For this review, take the finished solid that the model builds, in its own axes (mm). A direction names the side the tool comes from. Give positions to 0.01 mm unless a question says otherwise; leave off trailing zeros. Write each loop counter-clockwise with the first axis right and the second up, starting at its lowest first coordinate (ties: lowest second). Pieces come first, ordered by that corner, then holes. Notation, with made-up numbers: M 4,81 L 62,81 A17 cw 62,109 Z; hole C -38.5,-5.5 d8. An arc over 180 degrees is marked long. Answer as a JSON object with one key per item and string values. Group by question number.
```python
from build123d import *

# Parameters (mm, degrees)
SKETCH2_W                       = 25
SKETCH2_H                       = 130
SKETCH2_R                       = 5.1
SKETCH2_R_2                     = 7.5
BOSS_EXTRUDE1_DEPTH             = 6.35
TAP_DRILL_FOR_M3X0_5_TAP1_D     = 2.5
TAP_DRILL_FOR_M3X0_5_TAP1_DEPTH = 12.5
TAP_DRILL_FOR_M3X0_5_TAP1_TIP   = 0.751075774
BOSS_EXTRUDE2_DEPTH             = 6.35
F_1_4_CLEARANCE_HOLE1_D         = 6.7564
TAP_DRILL_FOR_M3X0_5_TAP2_D     = 2.5


with BuildPart() as part:
    # Sketch2 → Boss-Extrude1 (new body)
    with BuildSketch(Plane.XY):
        with Locations((0, 43.85)):
            Rectangle(SKETCH2_W, SKETCH2_H)
        Circle(SKETCH2_R, mode=Mode.SUBTRACT)
        with Locations((0, 25)):
            Circle(SKETCH2_R_2, mode=Mode.SUBTRACT)
        with Locations((0, 50)):
            Circle(SKETCH2_R_2, mode=Mode.SUBTRACT)
    extrude(amount=BOSS_EXTRUDE1_DEPTH)

    # Tap Drill for M3x0.5 Tap1
    with Locations(Plane.ZY.offset(12.5)):
        with Locations((3.175, 50), (3.175, 0), (3.175, 25)):
            Hole(TAP_DRILL_FOR_M3X0_5_TAP1_D / 2, depth=TAP_DRILL_FOR_M3X0_5_TAP1_DEPTH)
            with Locations((0, 0, -(TAP_DRILL_FOR_M3X0_5_TAP1_DEPTH + TAP_DRILL_FOR_M3X0_5_TAP1_TIP / 2))):  # 118° drill point
                Cone(0, TAP_DRILL_FOR_M3X0_5_TAP1_D / 2, TAP_DRILL_FOR_M3X0_5_TAP1_TIP, mode=Mode.SUBTRACT)

    # Sketch8 → Boss-Extrude2 (add)
    with BuildSketch(Plane(origin=(0, 0, 0), x_dir=(-1, 0, 0), z_dir=(0, 0, -1))):
        Polygon((12.5, 73.85), (22.5, 83.85), (22.5, 108.85), (12.5, 108.85), align=None)
    extrude(amount=-BOSS_EXTRUDE2_DEPTH)

    # 1/4 Clearance Hole1 (through all)
    with Locations(Plane.XY.offset(6.35)):
        with Locations((-12.5, 86.85), (-12.5, 100.85)):
            Hole(F_1_4_CLEARANCE_HOLE1_D / 2)

    # Tap Drill for M3x0.5 Tap2 (through all)
    with Locations(Plane.XY.offset(6.35)):
        with Locations((-8, 0), (0, 8), (8, 0), (0, -8)):
            Hole(TAP_DRILL_FOR_M3X0_5_TAP2_D / 2)


solid = part.part
```
Item 1: To check wall thickness, follow probe 1 along Y at (x, z) = (0, 3.5); probe 2 along Y at (x, z) = (-8, 1); probe 3 along Z at (x, y) = (-11, 0) (3 decimals). State the ranges of each line that lie inside material, in increasing order.
Item 2: Insertion check: P1, Ø6, axis at x = -12.5, y = 100.85, coming from the -Z side; P2, Ø1.5, axis at y = 4.5, z = 5.5, coming from the -X side. Each pin has a flat end and moves straight along its axis. Give the tip position at first contact, or say it passes through.
Item 3: Consider section C-C (y = 100.85). Give the boundary of the cut face in (x, z).
Item 4: Consider section D-D (y = -8). Give the boundary of the cut face in (x, z).
Item 5: Machinability: for faces 5 (the cylindrical face through (-10.718, 0.375, 1.983)), 6 (the flat face through (-17.43, 78.78, 3.13)), which of the approach directions +Z, -Z, +X, -X, +Y, -Y give a long, thin tool a straight path to every point of the face, cutting with its end or side? Answer none if there is none.
Item 6: Consider section B-B (x = 0). Give the boundary of the cut face in (y, z), plus the area to 3 significant figures.
Item 7: Draft analysis for pull direction Z (two halves, no side actions). For faces 1 (the cylindrical face through (-6.111, 0.375, 1.983)), 2 (the cylindrical face through (-9.91, 23.78, 3.45)), 3 (the flat face through (-1, 59, 6.35)), 4 (the cylindrical face through (0.27, 6.78, 3.13)), state which applies: released by +Z, released by -Z, zero draft, split by the parting line, or undercut.
Item 8: Consider section A-A (y = 50). Give the boundary of the cut face in (x, z) (3 decimals), plus the area to 3 significant figures.
Result set:
{
 "1": {"probe 1": "y = -21.15 to -9.25, -6.75 to -5.1, 5.1 to 6.75, 9.25 to 17.5, 32.5 to 42.5, 57.5 to 108.85", "probe 2": "y = -21.15 to -1.25, 1.25 to 108.85", "probe 3": "z = 0 to 1.925, 4.425 to 6.35"},
 "2": {"P1": "passes through", "P2": "stops at x = -12.5"},
 "3": {"outline": "M -22.5,0 L -15.88,0 L -15.88,6.35 L -22.5,6.35 Z; M -9.12,0 L 12.5,0 L 12.5,6.35 L -9.12,6.35 Z"},
 "4": {"outline": "M -12.5,0 L -1.25,0 L -1.25,6.35 L -12.5,6.35 Z; M 1.25,0 L 12.5,0 L 12.5,6.35 L 1.25,6.35 Z"},
 "5": {"face 5": "-X", "face 6": "+Z, -Z, -X, -Y"},
 "6": {"outline": "M -21.15,0 L -9.25,0 L -9.25,6.35 L -21.15,6.35 Z; M -6.75,0 L -5.1,0 L -5.1,6.35 L -6.75,6.35 Z; M 5.1,0 L 6.75,0 L 6.75,6.35 L 5.1,6.35 Z; M 9.25,0 L 17.5,0 L 17.5,6.35 L 9.25,6.35 Z; M 32.5,0 L 42.5,0 L 42.5,6.35 L 32.5,6.35 Z; M 57.5,0 L 108.85,0 L 108.85,6.35 L 57.5,6.35 Z", "area": "538 mm^2"},
 "7": {"face 1": "undercut", "face 2": "undercut", "face 3": "released by +Z", "face 4": "zero draft"},
 "8": {"outline": "M -12.5,0 L -7.5,0 L -7.5,1.925 L -12.5,1.925 Z; M -12.5,4.425 L -7.5,4.425 L -7.5,6.35 L -12.5,6.35 Z; M 7.5,0 L 12.5,0 L 12.5,6.35 L 7.5,6.35 Z", "area": "51.0 mm^2"}
}
